Geometry check sheet. Reference: drawing and pictorial views, mm from the part's lowest x, y, z. A direction names the side the tool comes from. Give positions to 0.01 mm unless a question says otherwise; leave off trailing zeros. Order: outer loops, then holes, each group sorted by start corner. A loop starts at its lowest first (then second) coordinate and runs counter-clockwise, first axis right, second up. Notation, with made-up numbers: M 12.25,6 L 33.25,6 A17 ccw 33.25,39 Z; hole C -31.75,14 d1. An arc over 180 degrees is marked long. Answer as a JSON object with one key per item and string values. Group by question number.
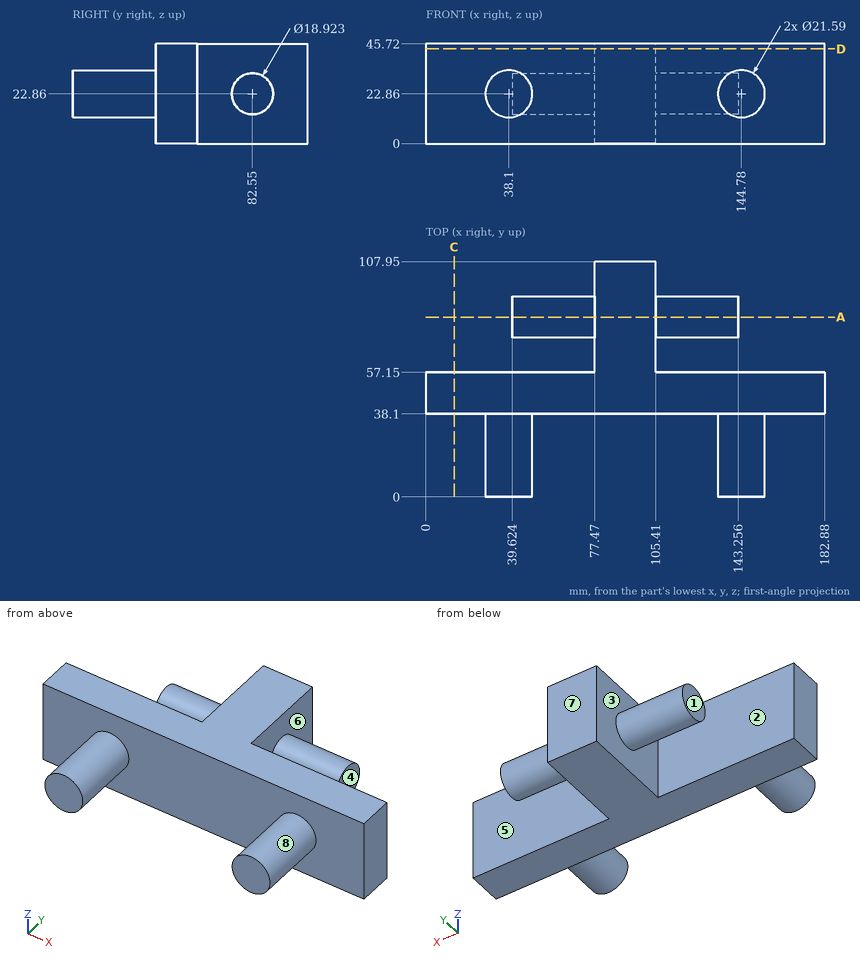
1. Release check for a two-part mould opening along X. For the marked faces 6, 7 and 8 record: released by +X, released by -X, zero draft, split by the parting line, or undercut.
2. Access from +Z, -Z, +X, -X, +Y, -Y to the whole of each face (thin tool, end or side, straight path). Record for the marked faces 1, 2, 3, 4 and 5.
3. Thickness scan on line 1 along Y through (x, z) = (141, 2); line 2 along X through (y, z) = (85.5, 6.5); line 3 along Y through (x, z) = (136, 17). Record the ranges inside material, lowest first. Write a range as [from, to].
4. Cross-section at C-C (x = 13). Record the cut outline in (y, z).
5. Depth check by flat-ended pin: pin 1 (6 mm diameter, centred on x = 112, z = 37.5, fed in from -Y); pin 2 (6 mm diameter, centred on x = 118, y = 86.5, fed in from -Z); pin 3 (13.5 mm diameter, centred on x = 40.5, z = 23, fed in from +Y); pin 4 (1 mm diameter, centred on x = 136, z = 29, fed in from -Y). Enter the tip coordinate at first touch or a pass-through.
6. Cross-section at D-D (z = 43.5). Record the cut outline in (x, y).
7. Cross-section at A-A (y = 82.55). Record the cut outline in (x, z).
Report:
{
 "1": {"face 6": "released by +X", "face 7": "zero draft", "face 8": "undercut"},
 "2": {"face 1": "+Z, -Z, -X, +Y", "face 2": "+Z, -Z, -X", "face 3": "-X", "face 4": "+Z, -Z, +X, +Y", "face 5": "+Z, -Z, +X"},
 "3": {"line 1": "y = [38.1, 57.15]", "line 2": "x = [77.47, 105.41]", "line 3": "y = [0, 57.15], [75.12, 89.98]"},
 "4": {"outline": "M 38.1,0 L 57.15,0 L 57.15,45.72 L 38.1,45.72 Z"},
 "5": {"pin 1": "stops at y = 38.1", "pin 2": "stops at z = 13.45", "pin 3": "stops at y = 92.01", "pin 4": "stops at y = 0"},
 "6": {"outline": "M 0,38.1 L 182.88,38.1 L 182.88,57.15 L 105.41,57.15 L 105.41,107.95 L 77.47,107.95 L 77.47,57.15 L 0,57.15 Z"},
 "7": {"outline": "M 39.62,13.4 L 77.47,13.4 L 77.47,0 L 105.41,0 L 105.41,13.4 L 143.26,13.4 L 143.26,32.32 L 105.41,32.32 L 105.41,45.72 L 77.47,45.72 L 77.47,32.32 L 39.62,32.32 Z"}
}
